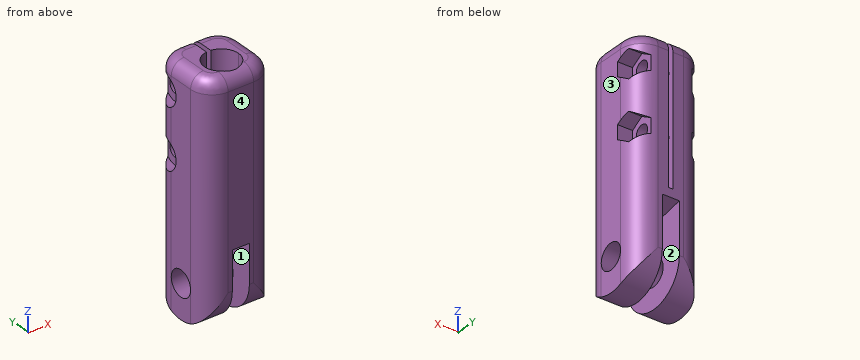
from build123d import *

# Parameters (mm, degrees)
SKETCH1_W               = 16
SKETCH1_H               = 16
BOSS_EXTRUDE1_DEPTH     = 55
SKETCH2_W               = 4
SKETCH2_H               = 17
CUT_EXTRUDE1_DEPTH      = 17
SKETCH3_R               = 3
CUT_EXTRUDE2_DEPTH      = 45
CUT_EXTRUDE3_DEPTH      = 33
FILLET1_R               = 5
FILLET2_R               = 3
CUT_EXTRUDE4_DEPTH      = 40
CUT_EXTRUDE4_DEPTH_BACK = 40
SKETCH5_R               = 1.75
CUT_EXTRUDE5_START      = -4
CUT_EXTRUDE5_DEPTH      = 40
CUT_EXTRUDE6_START      = -5
SKETCH7_R               = 3.5
CUT_EXTRUDE6_DEPTH      = 40
CUT_EXTRUDE7_DEPTH      = 58.835975073
CHAMFER1_SIZE2          = 16
CHAMFER1_SIZE           = 3


# Some blends are built 0.0001 mm under size
with BuildPart() as part:
    # Sketch1 → Boss-Extrude1 (new body)
    with BuildSketch(Plane.XY):
        Rectangle(SKETCH1_W, SKETCH1_H)
    extrude(amount=BOSS_EXTRUDE1_DEPTH)

    # Sketch2 → Cut-Extrude1 (cut)
    with BuildSketch(Plane(origin=(0, 8, 0), x_dir=(1, 0, 0), z_dir=(0, 1, 0))):
        with Locations((0, -8.5)):
            Rectangle(SKETCH2_W, SKETCH2_H)
    extrude(amount=-CUT_EXTRUDE1_DEPTH, mode=Mode.SUBTRACT)

    # Sketch3 → Cut-Extrude2 (cut)
    with BuildSketch(Plane(origin=(8, 0, 0), x_dir=(0, 0, -1), z_dir=(1, 0, 0))):
        with Locations((-8, 0)):
            Circle(SKETCH3_R)
    extrude(amount=-CUT_EXTRUDE2_DEPTH, mode=Mode.SUBTRACT)

    # Sketch4 → Cut-Extrude3 (cut)
    with BuildSketch(Plane.XY.offset(55)):
        with BuildLine():
            Line((0.5, 1.968626967), (0.5, 0.424558432))
            Line((0.5, 0.424558432), (-0.5, 0.424558432))
            Line((-0.5, 0.424558432), (-0.5, 1.968626967))
            ThreePointArc((-0.5, 1.968626967), (-2.645751311, -5), (4, -2))
            ThreePointArc((4, -2), (3, 0.645751311), (0.5, 1.968626967))
        make_face()
        with BuildLine():
            Line((-0.5, 0.424558432), (0.5, 0.424558432))
            Line((0.5, 0.424558432), (0.5, 1.968626967))
            ThreePointArc((0.5, 1.968626967), (0, 2), (-0.5, 1.968626967))
            Line((-0.5, 1.968626967), (-0.5, 0.424558432))
        make_face()
        with BuildLine():
            ThreePointArc((-0.5, 1.968626967), (0, 2), (0.5, 1.968626967))
            Line((0.5, 1.968626967), (0.5, 8))
            Line((0.5, 8), (-0.5, 8))
            Line((-0.5, 8), (-0.5, 1.968626967))
        make_face()
    extrude(amount=-CUT_EXTRUDE3_DEPTH, mode=Mode.SUBTRACT)

    # Fillet1
    fillet1_edges = [part.edges().sort_by_distance(p)[0] for p in [
        (8, -8, 27.5),
        (-8, -8, 27.5),
        (-8, 8, 27.5),
        (8, 8, 27.5),
    ]]
    fillet(fillet1_edges, radius=FILLET1_R - 0.0001)  # a hair under: the kernel refuses the full size

    # Fillet2
    # the kernel refuses this fillet: 3 mm, written as the material it takes off along each edge
    with BuildSketch(Plane(origin=(7, 8, 55), x_dir=(0, -1, 0), z_dir=(-1, 0, 0)), Plane(origin=(3.0001, 8, 55), x_dir=(0, -1, 0), z_dir=(-1, 0, 0))) as fillet2_piece_1:
        with BuildLine():
            CenterArc((FILLET2_R, -FILLET2_R), FILLET2_R, 90, 90)
            Line((0, -FILLET2_R), (0, 0))
            Line((0, 0), (FILLET2_R, 0))
        make_face()
    extrude(amount=10.0001, mode=Mode.SUBTRACT)
    with BuildSketch(Plane(origin=(8, -3.0001, 55), x_dir=(-1, 0, 0), z_dir=(0, 1, 0)), Plane(origin=(-8, 3.0001, 55), x_dir=(1, 0, 0), z_dir=(0, -1, 0))) as fillet2_piece_2:
        with BuildLine():
            CenterArc((FILLET2_R, -FILLET2_R), FILLET2_R, 90, 90)
            Line((0, -FILLET2_R), (0, 0))
            Line((0, 0), (FILLET2_R, 0))
        make_face()
    extrude(amount=6.0002, mode=Mode.SUBTRACT)
    with BuildSketch(Plane(origin=(-3.0001, -8, 55), x_dir=(0, 0, -1), z_dir=(1, 0, 0))) as fillet2_piece_3:
        with BuildLine():
            CenterArc((FILLET2_R, FILLET2_R), FILLET2_R, 180, 90)
            Line((0, FILLET2_R), (0, 0))
            Line((0, 0), (FILLET2_R, 0))
        make_face()
    extrude(amount=6.0002, mode=Mode.SUBTRACT)
    with BuildSketch(Plane(origin=(-3.0001, -3.0001, 55), x_dir=(0, -1, 0), z_dir=(1, 0, 0))) as fillet2_piece_4:
        with BuildLine():
            CenterArc((4.9999 - FILLET2_R, FILLET2_R), FILLET2_R, 270, 90)
            Line((4.9999 - FILLET2_R, 0), (4.9999, 0))
            Line((4.9999, 0), (4.9999, FILLET2_R))
        make_face()
    revolve(axis=Axis((-3.0001, -3.0001, 55), (0, 0, -1)), revolution_arc=90, mode=Mode.SUBTRACT)
    with BuildSketch(Plane(origin=(3.0001, -3.0001, 55), x_dir=(0, -1, 0), z_dir=(-1, 0, 0))) as fillet2_piece_5:
        with BuildLine():
            CenterArc((4.9999 - FILLET2_R, -FILLET2_R), FILLET2_R, 0, 90)
            Line((4.9999, -FILLET2_R), (4.9999, 0))
            Line((4.9999, 0), (4.9999 - FILLET2_R, 0))
        make_face()
    revolve(axis=Axis((3.0001, -3.0001, 55), (0, 0, 1)), revolution_arc=90, mode=Mode.SUBTRACT)
    with BuildSketch(Plane(origin=(-3.0001, 3.0001, 55), x_dir=(-1, 0, 0), z_dir=(0, -1, 0))) as fillet2_piece_6:
        with BuildLine():
            CenterArc((4.9999 - FILLET2_R, FILLET2_R), FILLET2_R, 270, 90)
            Line((4.9999, FILLET2_R), (4.9999, 0))
            Line((4.9999, 0), (4.9999 - FILLET2_R, 0))
        make_face()
    revolve(axis=Axis((-3.0001, 3.0001, 55), (0, 0, -1)), revolution_arc=90, mode=Mode.SUBTRACT)
    with BuildSketch(Plane(origin=(3.0001, 3.0001, 55), x_dir=(1, 0, 0), z_dir=(0, -1, 0))) as fillet2_piece_7:
        with BuildLine():
            CenterArc((4.9999 - FILLET2_R, -FILLET2_R), FILLET2_R, 0, 90)
            Line((4.9999, -FILLET2_R), (4.9999, 0))
            Line((4.9999, 0), (4.9999 - FILLET2_R, 0))
        make_face()
    revolve(axis=Axis((3.0001, 3.0001, 55), (0, 0, 1)), revolution_arc=90, mode=Mode.SUBTRACT)

    # Sketch5 → Cut-Extrude4 (cut, two sides: drawn at the far end of the back side and taken through both)
    with BuildSketch(Plane.ZY.offset(-0.5).offset(-CUT_EXTRUDE4_DEPTH_BACK)):
        with Locations(Location((48, 4.984313483, 0), (0, 0, 90))):
            Circle(SKETCH5_R)
        with Locations(Location((34, 4.984313483, 0), (0, 0, 90))):
            Circle(SKETCH5_R)
    extrude(amount=CUT_EXTRUDE4_DEPTH + CUT_EXTRUDE4_DEPTH_BACK, mode=Mode.SUBTRACT)

    # Sketch6 → Cut-Extrude5 (cut)
    with BuildSketch(Plane.ZY.offset(-0.5).offset(CUT_EXTRUDE5_START)):
        Polygon((49.674315781, 7.884313483), (46.325684219, 7.884313483), (44.651368439, 4.984313483), (46.325684219, 2.084313483), (49.674315781, 2.084313483), (51.348631561, 4.984313483), align=None)
        Polygon((35.885086056, 7.884313483), (32.536454495, 7.884313483), (30.862138714, 4.984313483), (32.536454495, 2.084313483), (35.885086056, 2.084313483), (37.559401836, 4.984313483), align=None)
    extrude(amount=-CUT_EXTRUDE5_DEPTH, mode=Mode.SUBTRACT)

    # Sketch7 → Cut-Extrude6 (cut)
    with BuildSketch(Plane(origin=(-0.5, 0, 0), x_dir=(0, 0, -1), z_dir=(1, 0, 0)).offset(CUT_EXTRUDE6_START)):
        with Locations((-48, 4.984313483)):
            Circle(SKETCH7_R)
        with Locations((-34, 4.984313483)):
            Circle(SKETCH7_R)
    extrude(amount=-CUT_EXTRUDE6_DEPTH, mode=Mode.SUBTRACT)

    # Sketch8 → Cut-Extrude7 (cut, through all)
    with BuildSketch(Plane.ZY.offset(8)):
        with BuildLine():
            Line((8, 8), (8.268392061, 14.01403494))
            ThreePointArc((8.268392061, 14.01403494), (-6.01403494, 0.268392061), (7.731607939, -14.01403494))
            Line((7.731607939, -14.01403494), (8, -8))
            ThreePointArc((8, -8), (0, 0), (8, 8))
        make_face()
    extrude(amount=-CUT_EXTRUDE7_DEPTH, mode=Mode.SUBTRACT)

    # Chamfer1
    chamfer1_edges = [part.edges().sort_by_distance(p)[0] for p in [
        (0, 8, 17),
    ]]
    chamfer1_side = [part.faces().sort_by_distance(p)[0] for p in [
        (0, 8, 17.06),
    ]]
    chamfer(chamfer1_edges, length=CHAMFER1_SIZE - 0.0001, length2=CHAMFER1_SIZE2 - 0.0001, reference=chamfer1_side[0])  # a hair under: the kernel refuses the full size


solid = part.part
The model under review builds one solid part; all positions refer to its coordinate system, in mm. Face numbers are marked on the shaded views. Give positions to 0.01 mm unless a question says otherwise; leave off trailing zeros. Order: outer loops, then holes, each group sorted by start corner. A loop starts at its lowest first (then second) coordinate and runs counter-clockwise, first axis right, second up. Notation, with made-up numbers: M -23.5,-18.75 L -7.5,-18.75 A29 ccw -7.5,5.25 Z; hole C 72,18 d6. An arc over 180 degrees is marked long. One line per question, with ' | ' between items. Start each with the question number.
1) Clearance check with flat-ended pins moving along their axes: P1, Ø3, axis at y = 4.98, z = 48, coming from the -X side; P2, Ø1, axis at x = -5.5, y = 1.5, coming from the -Z side; P3, Ø1.8, axis at y = 4.5, z = 36, coming from the +X side; P4, Ø4.5, axis at y = 5.5, z = 35.5, coming from the +X side. State where each tip first meets the part, or that it passes through.
2) Mouldability with a two-part tool opening along X and no side actions: class the marked faces 1, 2, 3 and 4 as pulls with the +X half, pulls with the -X half, needs draft (parallel to the pull), parting line crosses it, or undercut.
3) Consider section C-C, the plane y = -0.75. Give the boundary of the cut face in (x, z), then the cut area to 3 significant figures.
4) Consider section B-B, the plane z = 26. Give the boundary of the cut face in (x, y).
5) Consider section A-A, the plane z = 48. Give the boundary of the cut face in (x, y), then the cut area to 3 significant figures.
6) Wall thickness on L1, parallel to X at y = 2.5, z = 6; L2, parallel to X at y = -1.75, z = 27; L3, parallel to Z at x = -2.5, y = 4.5: over which ranges is each line inside the solid? List them lowest first. Write a range as from..to.
Found:
1) P1: passes through | P2: stops at z = 0.06 | P3: stops at x = 4.5 | P4: stops at x = 7.96
2) face 1: undercut | face 2: undercut | face 3: pulls with the +X half | face 4: needs draft
3) outline: M -8,0.04 L -2,0.04 L -2,5.1 L -8,5.1 Z; M -8,10.9 L -2,10.9 L -2,18.36 L 2,18.36 L 2,10.9 L 8,10.9 L 8,52 A3 ccw 5,55 L 3.8,55 L 3.8,22 L -3.8,22 L -3.8,55 L -5,55 A3 ccw -8,52 Z; M 2,0.04 L 8,0.04 L 8,5.1 L 2,5.1 Z | area: 482 mm²
4) outline: M -8,-3 A5 ccw -3,-8 L 3,-8 A5 ccw 8,-3 L 8,3 A5 ccw 3,8 L 0.5,8 L 0.5,1.97 A4 cw long -0.5,1.97 L -0.5,8 L -3,8 A5 ccw -8,3 Z
5) outline: M -8,-3 A5 ccw -3,-8 L 3,-8 A5 ccw 8,-3 L 8,2.08 L 4.5,2.08 L 4.5,3.23 L 0.5,3.23 L 0.5,1.97 A4 cw long -0.5,1.97 L -0.5,3.23 L -5.5,3.23 L -5.5,1.48 L -8,1.48 Z; M -5.5,6.73 L -0.5,6.73 L -0.5,8 L -3,8 A5 ccw -5.5,7.33 Z; M 0.5,6.73 L 4.5,6.73 L 4.5,7.77 A5 ccw 3,8 L 0.5,8 Z | area: 120 mm²
6) L1: x = -8..-2, 2..8 | L2: x = -8..-3.99, 3.99..8 | L3: z = 1.39..32.32, 35.68..46.32, 49.68..55
